Geometry check sheet. Reference: the model listing, model coordinates, mm. A direction names the side the tool comes from. Round coordinates to 2 decimals unless told otherwise and drop trailing zeros. Write each loop counter-clockwise with the first axis right and the second up, starting at its lowest first coordinate (ties: lowest second). Pieces come first, ordered by that corner, then holes. Notation, with made-up numbers: (-8.5, 85.5) -> (37.5, 85.5) arc R16 ccw to (37.5, 108.5) -> close; hole circle Ø6 at (89, 54). An arc over 180 degrees is marked (long way). Put each result on its own line as item: value. Start each with the question number.
from build123d import *

# Parameters (mm, degrees)
F1_DEPTH = 63.5
F3_DEPTH = 12.7
F4_R     = 13.783104
F5_DEPTH = 50.8


with BuildPart() as f1:
    # F0 (on Front) → F1 (new body)
    with BuildSketch(Plane.XZ):
        Polygon((6.323813, 37.759591), (-44.816598, 37.759591), (-44.816598, -51.69031), (67.362368, -51.69031), align=None)
    extrude(amount=F1_DEPTH)

    # F2 (on Front) → F3 (join)
    with BuildSketch(Plane.XZ):
        Polygon((-45.349181, 49.929906), (-45.0438, -51.151432), (74.971199, -51.151432), (7.481851, 49.929906), align=None)
    extrude(amount=F3_DEPTH)

    # F4 (on face) → F5 (cut)
    with BuildSketch(Plane(origin=(21.894957, 0, 14.940615), x_dir=(0, 1, 0), z_dir=(0.826012, 0, 0.563652))):
        with Locations((-38.936164, -18.272493)):
            Circle(F4_R)
    extrude(amount=-F5_DEPTH, mode=Mode.SUBTRACT)


solid = f1.part
(1) Sectioned sample at D-D (x = 44.5). Record the cut outline in (y, z).
(2) Material ranges on L1, parallel to Z at x = -12.5, y = -50; L2, parallel to Y at x = 53, z = -28.5; L3, parallel to Z at x = -1, y = -40, recorded low to high. Write a range as from..to.
(3) Set-up check for faces 4 (the flat face through (-19, -6, 49.93)), 5 (the flat face through (-19, -38, 37.76)): record each of +Z, -Z, +X, -X, +Y, -Y from which the full face is reachable in a straight line by a thin tool's end or side.
(4) Sectioned sample at B-B (x = -31). Record the cut outline in (y, z).
(5) Sectioned sample at A-A (y = -10.5). Record the cut outline in (x, z), and give its area (3 significant figures).
(6) Mould release check, pull along X, two halves, no side actions. Record for faces 1 (the flat face through (-9.876, -39.129, -28.627)), 2 (the flat face through (-2, -63.5, -16)), 3 (the flat face through (41.7, -6.26, -1.32)): +X half, -X half, draft (parallel to the pull), parting line (faces both ways), or undercut.
(7) Sectioned sample at C-C (y = -45.5). Record the cut outline in (x, z), and give its area (3 significant figures).
(8) Go/stop test with flat-tipped pins: pin 1 Ø3 at (y, z) = (-6.5, 5) entering from +X; pin 2 Ø8 at (y, z) = (-53.5, -2.5) entering from -X; pin 3 Ø4 at (y, z) = (-14, 26.5) entering from +X. Record where each tip stops, or that it passes through.
Found:
1. outline: (-63.5, -51.69) -> (0, -51.69) -> (0, -5.51) -> (-12.7, -5.51) -> (-12.7, -18.19) -> (-63.5, -18.19) -> close
2. L1: -51.69..-24.78, -20.7..37.76
2. L2: -12.7..0
2. L3: -51.69..-39.44, -6.17..37.76
3. face 4: +Z, +X, -X, +Y, -Y
3. face 5: +Z, +X, -X, -Y
4. outline: (-63.5, -51.69) -> (0, -51.69) -> (0, 49.93) -> (-12.7, 49.93) -> (-12.7, 37.76) -> (-63.5, 37.76) -> close
5. outline: (-45.35, 49.93) -> (-45.04, -51.15) -> (-44.82, -51.15) -> (-44.82, -51.69) -> (67.36, -51.69) -> (66.99, -51.15) -> (74.97, -51.15) -> (7.48, 49.93) -> close
5. area: 8,800 mm2
6. face 1: undercut
6. face 2: draft
6. face 3: +X half
7. outline: (-44.82, -51.69) -> (67.36, -51.69) -> (39.03, -10.16) -> (-2.94, -38.8) -> (-16.6, -18.78) -> (25.36, 9.86) -> (6.32, 37.76) -> (-44.82, 37.76) -> close
7. area: 6,070 mm2
8. pin 1: x = 38.48
8. pin 2: x = -44.82
8. pin 3: x = 24.14
